Check sheet for the modelled part. Datum: model origin and axes. Units: mm. Coordinates: 2 decimals unless noted, no trailing zeros. Loops run counter-clockwise (first coordinate to the right, second up) from the corner with the lowest first, then second, coordinate; pieces in that order, holes last.
```python
from build123d import *

# Parameters (mm, degrees)
SKETCH1_R           = 1.55
BOSS_EXTRUDE1_DEPTH = 1.5


with BuildPart() as part:
    # Sketch1 → Boss-Extrude1 (new body)
    with BuildSketch(Plane(origin=(0, 0, 0), x_dir=(1, 0, 0), z_dir=(0, 1, 0))):
        with BuildLine():
            Line((4.482e-06, 108.600000064), (4.482e-06, 5.000000064))
            ThreePointArc((4.482e-06, 5.000000064), (1.464470576, 1.464466159), (5.000004482, 6.4e-08))
            Line((5.000004482, 6.4e-08), (365.775004482, 6.4e-08))
            ThreePointArc((365.775004482, 6.4e-08), (369.310538388, 1.464466159), (370.775004482, 5.000000064))
            Line((370.775004482, 5.000000064), (370.775004482, 108.600000064))
            ThreePointArc((370.775004482, 108.600000064), (369.310538388, 112.13553397), (365.775004482, 113.600000064))
            Line((365.775004482, 113.600000064), (192.387504482, 113.600000064))
            Line((192.387504482, 113.600000064), (190.387504482, 111.600000064))
            Line((190.387504482, 111.600000064), (190.387504482, 104.600000064))
            Line((190.387504482, 104.600000064), (361.775004482, 104.600000064))
            Line((361.775004482, 104.600000064), (361.775004482, 9.000000064))
            Line((361.775004482, 9.000000064), (9.000004482, 9.000000064))
            Line((9.000004482, 9.000000064), (9.000004482, 104.600000064))
            Line((9.000004482, 104.600000064), (180.387504482, 104.600000064))
            Line((180.387504482, 104.600000064), (180.387504482, 111.600000064))
            Line((180.387504482, 111.600000064), (178.387504482, 113.600000064))
            Line((178.387504482, 113.600000064), (5.000004482, 113.600000064))
            ThreePointArc((5.000004482, 113.600000064), (1.464470576, 112.13553397), (4.482e-06, 108.600000064))
        make_face()
        with Locations(Location((195.387504482, 109.100000064, 0), (0, 0, 270))):
            Circle(SKETCH1_R, mode=Mode.SUBTRACT)
        with Locations(Location((175.387504482, 109.100000064, 0), (0, 0, 270))):
            Circle(SKETCH1_R, mode=Mode.SUBTRACT)
        with Locations(Location((85.387504482, 107.600000064, 0), (0, 0, 270))):
            Circle(SKETCH1_R, mode=Mode.SUBTRACT)
        with Locations(Location((285.387504482, 107.600000064, 0), (0, 0, 270))):
            Circle(SKETCH1_R, mode=Mode.SUBTRACT)
        with Locations(Location((85.387504482, 6.000000064, 0), (0, 0, 270))):
            Circle(SKETCH1_R, mode=Mode.SUBTRACT)
        with Locations(Location((185.387504482, 6.000000064, 0), (0, 0, 270))):
            Circle(SKETCH1_R, mode=Mode.SUBTRACT)
        with Locations(Location((285.387504482, 6.000000064, 0), (0, 0, 270))):
            Circle(SKETCH1_R, mode=Mode.SUBTRACT)
        Polygon((234.088466376, 111.350000064), (236.686542588, 111.350000064), (237.985580693, 109.100000064), (236.686542588, 106.850000064), (234.088466376, 106.850000064), (232.789428271, 109.100000064), align=None, mode=Mode.SUBTRACT)
        Polygon((334.088466376, 111.350000064), (336.686542588, 111.350000064), (337.985580693, 109.100000064), (336.686542588, 106.850000064), (334.088466376, 106.850000064), (332.789428271, 109.100000064), align=None, mode=Mode.SUBTRACT)
        Polygon((365.947436086, 110.609548976), (367.784553393, 108.772431669), (367.112121789, 106.262882757), (364.602572878, 105.590451153), (362.765455571, 107.42756846), (363.437887175, 109.937117372), align=None, mode=Mode.SUBTRACT)
        Polygon((136.686542588, 111.350000064), (134.088466376, 111.350000064), (132.789428271, 109.100000064), (134.088466376, 106.850000064), (136.686542588, 106.850000064), (137.985580693, 109.100000064), align=None, mode=Mode.SUBTRACT)
        Polygon((36.686542588, 111.350000064), (34.088466376, 111.350000064), (32.789428271, 109.100000064), (34.088466376, 106.850000064), (36.686542588, 106.850000064), (37.985580693, 109.100000064), align=None, mode=Mode.SUBTRACT)
        Polygon((4.827572878, 110.609548976), (2.990455571, 108.772431669), (3.662887175, 106.262882757), (6.172436086, 105.590451153), (8.009553393, 107.42756846), (7.337121789, 109.937117372), align=None, mode=Mode.SUBTRACT)
        Polygon((234.088466376, 2.250000064), (236.686542588, 2.250000064), (237.985580693, 4.500000064), (236.686542588, 6.750000064), (234.088466376, 6.750000064), (232.789428271, 4.500000064), align=None, mode=Mode.SUBTRACT)
        Polygon((334.088466376, 2.250000064), (336.686542588, 2.250000064), (337.985580693, 4.500000064), (336.686542588, 6.750000064), (334.088466376, 6.750000064), (332.789428271, 4.500000064), align=None, mode=Mode.SUBTRACT)
        Polygon((365.947436086, 2.990451153), (367.784553393, 4.82756846), (367.112121789, 7.337117372), (364.602572878, 8.009548976), (362.765455571, 6.172431669), (363.437887175, 3.662882757), align=None, mode=Mode.SUBTRACT)
        Polygon((136.686542588, 2.250000064), (134.088466376, 2.250000064), (132.789428271, 4.500000064), (134.088466376, 6.750000064), (136.686542588, 6.750000064), (137.985580693, 4.500000064), align=None, mode=Mode.SUBTRACT)
        Polygon((36.686542588, 2.250000064), (34.088466376, 2.250000064), (32.789428271, 4.500000064), (34.088466376, 6.750000064), (36.686542588, 6.750000064), (37.985580693, 4.500000064), align=None, mode=Mode.SUBTRACT)
        Polygon((4.827572878, 2.990451153), (2.990455571, 4.82756846), (3.662887175, 7.337117372), (6.172436086, 8.009548976), (8.009553393, 6.172431669), (7.337121789, 3.662882757), align=None, mode=Mode.SUBTRACT)
    extrude(amount=-BOSS_EXTRUDE1_DEPTH)


solid = part.part
```
1) Depth check by flat-ended pin: pin 1 (2.5 mm diameter, centred on x = 185.39, z = -6, fed in from +Y). Enter the tip coordinate at first touch or a pass-through.
Answer sheet:
pin 1: passes through
2) Section check A-A on x = 114.5. Enter the section's corners in (y, z).
Answer sheet:
outline: (-1.5, -113.6) - (0, -113.6) - (0, -104.6) - (-1.5, -104.6) - close; (-1.5, -9) - (0, -9) - (0, 0) - (-1.5, 0) - close
3) Section check B-B on z = -65.5. Enter the section's corners in (x, y) (3 decimals), plus the area to 3 significant figures.
Answer sheet:
outline: (0, -1.5) - (9, -1.5) - (9, 0) - (0, 0) - close; (361.775, -1.5) - (370.775, -1.5) - (370.775, 0) - (361.775, 0) - close
area: 27.0 mm2
4) Scan lines: line 1 (Z direction, x = 96, y = -1.35); line 2 (X direction, y = -0.3, z = -19) (3 decimals). Record each from-to range of solid material in increasing order.
Answer sheet:
line 1: z = -113.6 to -104.6, -9 to 0
line 2: x = 0 to 9, 361.775 to 370.775
5) Section check C-C on y = -1. Give the number of separate pieces and of enclosed holes in the cut face, plus the area to 3 significant figures.
Answer sheet:
separate pieces: 1
enclosed holes: 19
area: 8,020 mm2
